Input: part model. Units: mm. Frame: model coordinates. Face numbers are marked on the shaded views. A direction names the side the tool comes from. Coordinates: 2 decimals unless noted, no trailing zeros. Write each loop counter-clockwise with the first axis right and the second up, starting at its lowest first coordinate (ties: lowest second). Pieces come first, ordered by that corner, then holes.
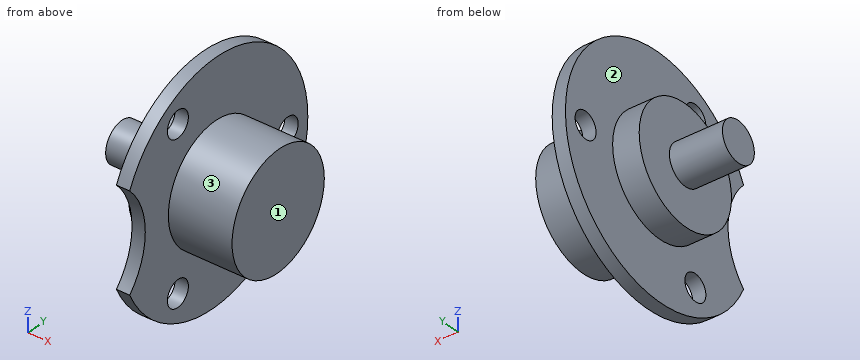
Autodesk Inventor part; units mm, degrees
ref_plane "YZ Plane" through (0, 0, 0) normal (1, 0, 0) x (0, 1, 0)
ref_plane "XZ Plane" through (0, 0, 0) normal (0, 1, 0) x (-1, 0, 0)
ref_plane "XY Plane" through (0, 0, 0) normal (0, 0, 1) x (1, 0, 0)
sketch "Sketch1" plane through (0, 0, 0) normal (0, 0, 1) x (1, 0, 0)
  line L0 (0, 0) -> (0, 3.8)
  line L1 (0, 3.8) -> (0, 3.8)
  line L2 (0, 3.8) -> (0, 11)
  line L3 (0, 11) -> (5, 11)
  line L4 (5, 11) -> (5, 22.25)
  line L5 (5, 22.25) -> (7.5, 22.25)
  line L6 (7.5, 22.25) -> (7.5, 11)
  line L7 (7.5, 11) -> (19.5, 11)
  line L8 (19.5, 11) -> (19.5, 0)
  line L9 (19.5, 0) -> (0, 0)
  line L10 (0, 0) -> (41.6069, 0)
  dimension "d0" = 7.6
  dimension "d1" = 22
  dimension "d2" = 44.5
  dimension "d3" = 0
  dimension "d4" = 5
  dimension "d5" = 12
  dimension "d6" = 2.5
revolve "Revolution1" add sketch "Sketch1" angle 360 about axis through (0, 0, 0) along (1, 0, 0)
sketch "Sketch2" plane through (0, 0, 0) normal (-1, 0, 0) x (0, 0, 1)
  circle A0 centre (0, 0) radius 11
  circle A1 centre (0, 0) radius 3.8
  dimension "d8" = 7.6
extrude "Extrusion1" add sketch "Sketch2" along normal blind 10 contours A1
sketch "Sketch3" plane through (7.5, 0, 0) normal (1, 0, 0) x (0, 0, -1)
  circle A0 centre (0, 0) radius 22.25
  circle A1 centre (0, 17.45) radius 2.5
  circle A2 centre (15.1121, -8.725) radius 2.5
  circle A3 centre (-15.1121, -8.725) radius 2.5
  line L0 (0, 0) -> (0, 17.45) construction
  line L1 (0, 0) -> (15.1121, -8.725) construction
  line L2 (0, 0) -> (-15.1121, -8.725) construction
  dimension "d11" = 5
  dimension "d12" = 17.45
  dimension "d13" = 17.45
  dimension "d14" = 17.45
  dimension "d15" = 5
  dimension "d16" = 5
  dimension "d17" = 120
  dimension "d18" = 120
extrude "Extrusion2" cut sketch "Sketch3" against normal through all contours A1 | A2 | A3
sketch "Sketch4" plane through (7.5, 0, 0) normal (1, 0, 0) x (0, 0, -1)
  circle A0 centre (0, 0) radius 11
  circle A1 centre (0, 0) radius 22.25
  arc A2 (9.2992, -20.2135) -> (-9.2992, -20.2135) centre (0, -30) ccw
  dimension "d21" = 13.5
  dimension "d22" = 30
extrude "Extrusion3" cut sketch "Sketch4" against normal through all contours A2 A1 picked at (-2.0741, -20.1881)
properties part number "Släpring"
Item 1: Section query D-D, the plane x = 11.25. Return loops of the section in (y, z), then the cut area to 3 significant figures.
Item 2: Access query for the marked faces 1, 2 and 3. Directions: +Z, -Z, +X, -X, +Y, -Y. A direction counts if a zero-diameter tool reaches every point of the face in a straight line with its end or side. Return the directions, or none.
Item 3: Material intervals for line 1 (X direction, y = -14.5, z = 16.5); line 2 (Z direction, x = 1.5, y = 0); line 3 (X direction, y = -1, z = 8.5), sorted ascending.
Item 4: Section query B-B, the plane y = 0. Return loops of the section in (x, z), then the cut area to 3 significant figures.
Item 5: Section query A-A, the plane z = 0. Return loops of the section in (x, y).
Item 6: Section query C-C, the plane y = 17.45. Return loops of the section in (x, z), then the cut area to 3 significant figures.
Item 7: Pin query (flat end, axial travel): pin 1 Ø2 at (x, z) = (3.5, -1.5) entering from +Y; pin 2 Ø8 at (x, z) = (10.5, 17) entering from -Y; pin 3 Ø8 at (y, z) = (0, 15.5) entering from -X; pin 4 Ø17.5 at (y, z) = (3, -3) entering from -X. Return the tip coordinate at first contact, or that it passes through.
The answers:
1. outline: circle Ø22 at (0, 0)
1. area: 380 mm2
2. face 1: +Z, -Z, +X, +Y, -Y
2. face 2: -X
2. face 3: +X
3. line 1: x = 5 to 7.5
3. line 2: z = -11 to 11
3. line 3: x = 0 to 19.5
4. outline: (-10, -3.8) - (0, -3.8) - (0, -11) - (5, -11) - (5, -22.25) - (7.5, -22.25) - (7.5, -11) - (19.5, -11) - (19.5, 11) - (7.5, 11) - (7.5, 22.25) - (5, 22.25) - (5, 11) - (0, 11) - (0, 3.8) - (-10, 3.8) - close
4. area: 561 mm2
5. outline: (-10, -3.8) - (0, -3.8) - (0, -11) - (5, -11) - (5, -16.5) - (7.5, -16.5) - (7.5, -11) - (19.5, -11) - (19.5, 11) - (7.5, 11) - (7.5, 14.95) - (5, 14.95) - (5, 11) - (0, 11) - (0, 3.8) - (-10, 3.8) - close; (5, 19.95) - (7.5, 19.95) - (7.5, 22.25) - (5, 22.25) - close
6. outline: (5, -13.8) - (7.5, -13.8) - (7.5, -2.5) - (5, -2.5) - close; (5, 2.5) - (7.5, 2.5) - (7.5, 13.8) - (5, 13.8) - close
6. area: 56.5 mm2
7. pin 1: stops at y = 10.99
7. pin 2: stops at y = -17
7. pin 3: stops at x = 5
7. pin 4: stops at x = -10
